The listing builds one solid part. Answer for the finished solid, in the listing's coordinates (mm). Face numbers are marked on the shaded views. A direction names the side the tool comes from. Give positions to 0.01 mm unless a question says otherwise; leave off trailing zeros. Order: outer loops, then holes, each group sorted by start corner. A loop starts at its lowest first (then second) coordinate and runs counter-clockwise, first axis right, second up.
```python
from build123d import *

# Parameters (mm, degrees)
F0_R     = 56.6410557647
F1_DEPTH = 414.35633
F2_R     = 56.6410557647
F3_DEPTH = 25.4
F4_R     = 56.6410557647
F5_DEPTH = 638.01814
F5_TAPER = 6
F6_R     = 56.6410557647
F7_DEPTH = 443.62
F8_R     = 56.6410557647
F9_DEPTH = 335.84362
F9_TAPER = -8


with BuildPart() as f1:
    # F0 (on Top) → F1 (new body)
    with BuildSketch(Plane.XY):
        Circle(F0_R)
    extrude(amount=-F1_DEPTH)

    # F2 (on face) → F3 (join)
    with BuildSketch(Plane.XY):
        Circle(F2_R)
    extrude(amount=F3_DEPTH)

    # F4 (on face) → F5 (join)
    with BuildSketch(Plane.XY.offset(25.4)):
        Circle(F4_R)
    extrude(amount=F5_DEPTH, taper=F5_TAPER)

    # F6 (on face) → F7 (join)
    with BuildSketch(Plane(origin=(0, 0, -414.35633), x_dir=(1, 0, 0), z_dir=(0, 0, -1))):
        Circle(F6_R)
    extrude(amount=F7_DEPTH)

    # F8 (on face) → F9 (join)
    with BuildSketch(Plane(origin=(0, 0, -857.97633), x_dir=(1, 0, 0), z_dir=(0, 0, -1))):
        Circle(F8_R)
    extrude(amount=F9_DEPTH, taper=F9_TAPER)


solid = f1.part
```
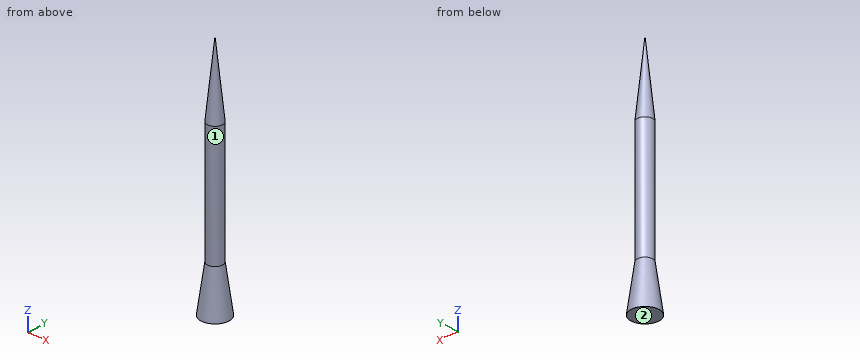
1) A tool of negligible diameter and unlimited length cuts with its end or side. For the marked faces 1 and 2, from which of +Z, -Z, +X, -X, +Y, -Y can it reach the whole face along a straight path? Write none if from no direction.
Geometry says:
face 1: +Z
face 2: -Z, +X, -X, +Y, -Y
2) Given P1, Ø6, axis at x = -53.5, z = -530, coming from the -Y side; P2, Ø6, axis at x = -5, z = -164, coming from the -Y side; P3, Ø6, axis at y = 11, z = -659, coming from the -X side, each flat-ended and moving along its own axis, determine where each tip first touches the part or whether it passes through.
Geometry says:
P1: stops at y = -25.65
P2: stops at y = -56.61
P3: stops at x = -56.07
3) Straight lines are drawn through the part: probe 1 along X at (y, z) = (-5.5, -745.5); probe 2 along X at (y, z) = (37.5, 139); probe 3 along Y at (x, z) = (40.5, -716). For each, find the intervals that lie inside material, in ascending order.
Geometry says:
probe 1: x = -56.37 to 56.37
probe 2: x = -24.33 to 24.33
probe 3: y = -39.6 to 39.6
4) Find section A-A (z = -422). Write down the section's boundary in (x, y), then the cut area to 3 significant figures.
Geometry says:
outline: circle Ø113.28 at (0, 0)
area: 10,100 mm2
5) Find section B-B (z = -956.5). Write down the section's boundary in (x, y), then the cut area to 3 significant figures.
Geometry says:
outline: circle Ø140.98 at (0, 0)
area: 15,600 mm2
